Source: three-view drawing plus pictorial views. Frame: mm from the lowest corner of the part. Give positions to 0.01 mm unless a question says otherwise; leave off trailing zeros. Loops run counter-clockwise (first coordinate to the right, second up) from the corner with the lowest first, then second, coordinate; pieces in that order, holes last. Notation, with made-up numbers: (25, 50) - (60, 50) arc R7 cw to (60, 61) - close; hole circle Ø8 at (82.5, -39.75). An arc over 180 degrees is marked (long way). Answer in a Markdown table with one row per item.
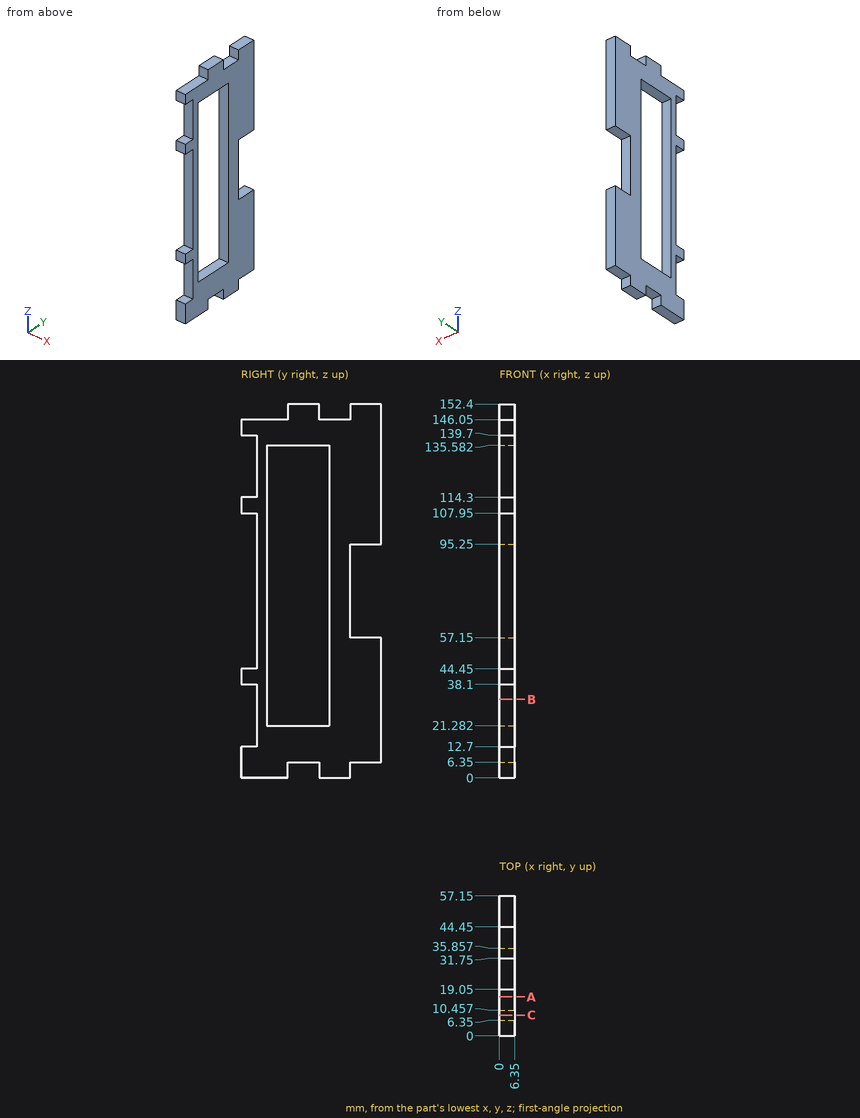
Q1. Cut plane B-B (z = 32). Output: boundary loops of the cut face in (x, y).
Check values:
| item | result |
|---|---|
| outline | (0, 6.35) - (6.35, 6.35) - (6.35, 10.46) - (0, 10.46) - close; (0, 35.86) - (6.35, 35.86) - (6.35, 57.15) - (0, 57.15) - close |
Q2. Cut plane C-C (y = 8.5). Output: boundary loops of the cut face in (x, z).
Check values:
| item | result |
|---|---|
| outline | (0, 0) - (6.35, 0) - (6.35, 146.05) - (0, 146.05) - close |
Q3. Material intervals for line 1 along Z through (x, y) = (6, 3); line 2 along Y through (x, z) = (2.5, 49); line 3 along Z through (x, y) = (6.25, 16), sorted ascending.
Check values:
| item | result |
|---|---|
| line 1 | 0 to 12.7, 38.1 to 44.45, 107.95 to 114.3, 139.7 to 146.05 |
| line 2 | 6.35 to 10.46, 35.86 to 57.15 |
| line 3 | 0 to 21.28, 135.58 to 146.05 |
Q4. Cut plane A-A (y = 16). Output: boundary loops of the cut face in (x, z), and give its area (3 significant figures).
Check values:
| item | result |
|---|---|
| outline | (0, 0) - (6.35, 0) - (6.35, 21.28) - (0, 21.28) - close; (0, 135.58) - (6.35, 135.58) - (6.35, 146.05) - (0, 146.05) - close |
| area | 202 mm² |
Q5. First-contact query: pin 1 (1.9 mm diameter, centred on x = 2.5, y = 4.5, fed in from +Z); pin 2 (1.9 mm diameter, centred on x = 2, z = 150.5, fed in from -Y); pin 3 (3 mm diameter, centred on x = 4.5, y = 48, fed in from -Z). Flat tips, straight axial feed; report the tip coordinate or a pass-through.
Check values:
| item | result |
|---|---|
| pin 1 | z = 146.05 |
| pin 2 | y = 19.05 |
| pin 3 | z = 6.35 |
